Geometry: final body of the model. Coordinates: model frame, mm. Face numbers are marked on the shaded views. A direction names the side the tool comes from. Give positions to 0.01 mm unless a question says otherwise; leave off trailing zeros. Loops run counter-clockwise (first coordinate to the right, second up) from the corner with the lowest first, then second, coordinate; pieces in that order, holes last.
1. Material intervals for line 1 along Y through (x, z) = (0, 19.1) (3 decimals); line 2 along Y through (x, z) = (0, 5.6); line 3 along Y through (x, z) = (0, 9), sorted ascending.
2. Section B-B, the plane z = 22.75. Output: boundary loops of the cut face in (x, y), then the cut area to 3 significant figures.
3. Section A-A, the plane z = 7.75. Output: boundary loops of the cut face in (x, y), then the cut area to 3 significant figures.
4. First-contact query: P1, Ø4, axis at x = 7.5, y = 6, coming from the -Z side; P2, Ø2, axis at y = -6.5, z = 24.5, coming from the -X side; P3, Ø6, axis at y = -5, z = 10.5, coming from the +X side; P4, Ø9.5, axis at x = -1.5, y = -1.5, coming from the -Z side. Flat tips, straight axial feed; report the tip coordinate or a pass-through.
5. Draft query along X for the marked faces 1, 2 and 3. Return one class per face: +X half, -X half, draft (parallel to the pull), parting line (faces both ways), or undercut.
6. Access query for the marked faces 4 and 5. Directions: +Z, -Z, +X, -X, +Y, -Y. A direction counts if a zero-diameter tool reaches every point of the face in a straight line with its end or side. Return the directions, or none.
7. Section C-C, the plane z = 17.5. Output: boundary loops of the cut face in (x, y) (3 decimals).
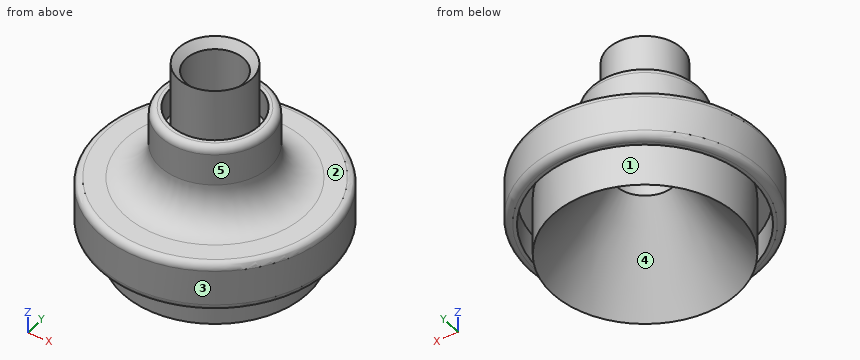
from build123d import *

# Parameters (mm, degrees)
FILLET_R    = 1
FILLET001_R = 1
FILLET002_R = 1


with BuildPart() as part:
    # Sketch → Revolution (revolve)
    with BuildSketch(Plane.XZ):
        with BuildLine():
            Line((4.1, 27.4), (4.1, 12))
            Line((4.1, 12), (13.15, 0))
            Line((13.15, 0), (13.15, 8.5))
            Line((13.15, 8.5), (15, 8.5))
            Line((15, 8.5), (15, 4.5))
            Line((15, 4.5), (16.5, 4.5))
            Line((16.5, 4.5), (16.5, 11.5))
            Line((16.5, 11.5), (12.775, 11.5))
            ThreePointArc((7.775, 16.5), (9.239466, 12.964466), (12.775, 11.5))
            Line((7.775, 22), (7.775, 16.5))
            Line((6.275, 22), (7.775, 22))
            Line((6.275, 18), (6.275, 22))
            Line((5.2, 18), (6.275, 18))
            Line((5.2, 28.5), (5.2, 18))
            Line((4.1, 27.4), (5.2, 28.5))
        make_face()
    revolve(axis=Axis((0, 0, 0), (0, 0, 1)))

    # Fillet
    fillet_edges = [part.edges().sort_by_distance(p)[0] for p in [
        (-16.5, 0, 4.5),
    ]]
    fillet(fillet_edges, radius=FILLET_R)

    # Fillet001
    fillet001_edges = [part.edges().sort_by_distance(p)[0] for p in [
        (-16.5, 0, 11.5),
    ]]
    fillet(fillet001_edges, radius=FILLET001_R)

    # Fillet002
    fillet002_edges = [part.edges().sort_by_distance(p)[0] for p in [
        (-7.775, 0, 22),
    ]]
    fillet(fillet002_edges, radius=FILLET002_R)


solid = part.part
Answers below:
1. line 1: y = -7.775 to -6.275, -5.2 to -4.1, 4.1 to 5.2, 6.275 to 7.775
1. line 2: y = -16.5 to -15, -13.15 to -8.93, 8.93 to 13.15, 15 to 16.5
1. line 3: y = -16.5 to -6.36, 6.36 to 16.5
2. outline: circle Ø10.4 at (0, 0); hole circle Ø8.2 at (0, 0)
2. area: 32.1 mm2
3. outline: circle Ø33 at (0, 0); circle Ø26.3 at (0, 0); hole circle Ø30 at (0, 0); hole circle Ø14.61 at (0, 0)
3. area: 524 mm2
4. P1: stops at z = 2.05
4. P2: passes through
4. P3: stops at x = 16.38
4. P4: stops at z = 8.33
5. face 1: undercut
5. face 2: draft
5. face 3: parting line
6. face 4: -Z
6. face 5: +Z
7. outline: circle Ø15.55 at (0, 0); hole circle Ø8.2 at (0, 0)
